Input: part model. Units: mm. Frame: model coordinates. A direction names the side the tool comes from. Coordinates: 2 decimals unless noted, no trailing zeros. Order: outer loops, then holes, each group sorted by start corner. A loop starts at its lowest first (then second) coordinate and runs counter-clockwise, first axis right, second up. Notation, with made-up numbers: (42.25, -18) -> (61.25, -18) arc R36 ccw to (61.25, 18) -> close; hole circle Ø1 at (-11, 39.5). An arc over 180 degrees is marked (long way). Answer as CSV lines item,"result".
from build123d import *

# Parameters (mm, degrees)
SKETCH_1_R      = 35
SKETCH_1_R_2    = 27.5
EXTRUDE_1_DEPTH = 60
CHAMFER_1_SIZE  = 3
SKETCH_2_W      = 29
SKETCH_2_H      = 2.2
CHAMFER_2_SIZE  = 1


with BuildPart() as part:
    # 草图1 → 凸台-拉伸1 (new body)
    with BuildSketch(Plane.XY):
        Circle(SKETCH_1_R)
        Circle(SKETCH_1_R_2, mode=Mode.SUBTRACT)
    extrude(amount=EXTRUDE_1_DEPTH)

    # 倒角1
    chamfer_1_edges = [part.edges().sort_by_distance(p)[0] for p in [
        (-35, 0, 0),
        (-35, 0, 60),
    ]]
    chamfer(chamfer_1_edges, length=CHAMFER_1_SIZE)

    # 草图2 → 切除-旋转1 (revolve, cut)
    with BuildSketch(Plane(origin=(0, 0, 0), x_dir=(1, 0, 0), z_dir=(0, 1, 0)), mode=Mode.PRIVATE) as cut_revolve_1_sk:
        with Locations((14.5, -5.6)):
            Rectangle(SKETCH_2_W, SKETCH_2_H)
    revolve(cut_revolve_1_sk.sketch.rotate(Axis((0, 0, 0), (0, 0, 1)), 180), axis=Axis((0, 0, 0), (0, 0, 1)), mode=Mode.SUBTRACT)

    # 倒角2
    chamfer_2_edges = [part.edges().sort_by_distance(p)[0] for p in [
        (-27.5, 0, 0),
        (-27.5, 0, 60),
    ]]
    chamfer(chamfer_2_edges, length=CHAMFER_2_SIZE)


solid = part.part
1. Mould query, pull axis Z, two halves, no side actions, for faces 1 (the face through (-13.38, 25.73, 5.58)), 2 (the face through (-32.115, 1.413, 59.854)), 3 (the face through (-28, -21, 30)), 4 (the face through (17, -22, 6.7)). Classes: released by +Z, released by -Z, zero draft, split by the parting line, or undercut.
Findings:
face 1,"undercut"
face 2,"released by +Z"
face 3,"zero draft"
face 4,"undercut"
2. Ray query, line 1 along Y through (x, z) = (0, 26.5); line 2 along Y through (x, z) = (0, 5.95); line 3 along X through (y, z) = (0, 2). Return the intervals inside material, ascending.
Findings:
line 1,"y = -35 to -27.5, 27.5 to 35"
line 2,"y = -35 to -29, 29 to 35"
line 3,"x = -34 to -27.5, 27.5 to 34"
3. Contact query for flat-ended pins moving along their axis: pin 1 (2 mm diameter, centred on x = 23.5, z = 20.5, fed in from +Y); pin 2 (3 mm diameter, centred on y = 9, z = 43.5, fed in from -X); pin 3 (12 mm diameter, centred on y = -9.5, z = 7, fed in from -X). Output: stop coordinate, or through.
Findings:
pin 1,"stops at y = 26.81"
pin 2,"stops at x = -34.19"
pin 3,"stops at x = -34.82"
4. Reachability of faces 5 (the face through (17, -22, 4.5)), 6 (the face through (-32.115, 1.413, 0.146)) from +Z, -Z, +X, -X, +Y, -Y: full face, straight path, thin tool, end or side. Return the list, or none.
Findings:
face 5,"none"
face 6,"-Z"
5. Cut plane A-A (x = 0). Return the cut outline in (y, z), plus the area to 3 significant figures.
Findings:
outline,"(-35, 3) -> (-32, 0) -> (-28.5, 0) -> (-27.5, 1) -> (-27.5, 4.5) -> (-29, 4.5) -> (-29, 6.7) -> (-27.5, 6.7) -> (-27.5, 59) -> (-28.5, 60) -> (-32, 60) -> (-35, 57) -> close; (27.5, 1) -> (28.5, 0) -> (32, 0) -> (35, 3) -> (35, 57) -> (32, 60) -> (28.5, 60) -> (27.5, 59) -> (27.5, 6.7) -> (29, 6.7) -> (29, 4.5) -> (27.5, 4.5) -> close"
area,"873 mm2"
6. Cut plane C-C (z = 35.5). Return the cut outline in (x, y).
Findings:
outline,"circle Ø70 at (0, 0); hole circle Ø55 at (0, 0)"
